Autodesk Inventor part; units mm, degrees
ref_plane "YZ Plane" through (0, 0, 0) normal (1, 0, 0) x (0, 1, 0)
ref_plane "XZ Plane" through (0, 0, 0) normal (0, 1, 0) x (-1, 0, 0)
ref_plane "XY Plane" through (0, 0, 0) normal (0, 0, 1) x (1, 0, 0)
sketch "Sketch1" plane through (0, 0, 0) normal (0, 0, 1) x (1, 0, 0)
  line L0 (-9, -62.5) -> (9, -62.5)
  line L1 (9, -62.5) -> (9, 62.5)
  line L2 (9, 62.5) -> (-9, 62.5)
  line L3 (-9, 62.5) -> (-9, -62.5)
  line L4 (-9, -62.5) -> (9, 62.5) construction
  line L5 (9, -62.5) -> (-9, 62.5) construction
  point P0 (0, 0)
  dimension "d0" = 18
  dimension "d1" = 125
extrude "Plate1" add sketch "Sketch1" along normal blind 2
sketch "Sketch2" plane through (-9, 60.5, 0) normal (0, 1, 0) x (-1, 0, 0)
  line L0 (-18, 0) -> (0, 0)
  line L1 (0, 0) -> (0, 25)
  line L2 (0, 25) -> (-18, 25)
  line L3 (-18, 25) -> (-18, 0)
edge flange "Flange1" height 25 angle 90 thickness 2 bend radius 2 thickness toward (0, 1, 0) relief tear relief width 2 relief depth 1 edges at (0, 62.5, 2) wall of the first edge with corners at (9, 60.5, 0) (-9, 60.5, 0) (-9, 60.5, 25) (9, 60.5, 25)
bend "Bend1"
corner "Corner1"
sketch "Sketch3" plane through (0, 0, 2) normal (0, 0, 1) x (1, 0, 0)
  line L0 (-1.75, -57.5) -> (1.75, -57.5) construction
  line L1 (-1.75, -59.2) -> (1.75, -59.2)
  line L2 (1.75, -55.8) -> (-1.75, -55.8)
  arc A0 (-1.75, -55.8) -> (-1.75, -59.2) centre (-1.75, -57.5) ccw
  arc A1 (1.75, -59.2) -> (1.75, -55.8) centre (1.75, -57.5) ccw
  line L3 (-1.75, 36.5) -> (1.75, 36.5) construction
  line L4 (-9, -62.5) -> (-9, 58.5)
  line L5 (-1.75, 34.8) -> (1.75, 34.8)
  line L6 (1.75, 38.2) -> (-1.75, 38.2)
  arc A2 (-1.75, 38.2) -> (-1.75, 34.8) centre (-1.75, 36.5) ccw
  arc A3 (1.75, 34.8) -> (1.75, 38.2) centre (1.75, 36.5) ccw
  line L7 (9, -62.5) -> (-9, -62.5)
  point P0 (0, 0)
  point P1 (0, -57.5)
  point P2 (0, 36.5)
  dimension "d13" = 94
  dimension "d14" = 5
  dimension "d15" = 3.4
  dimension "d16" = 3.5
extrude "Cut1" cut sketch "Sketch3" against normal blind 2
sketch "Sketch4" plane through (-9, 62.5, 25) normal (0, 1, 0) x (1, 0, 0)
  line L0 (12, 10.5) -> (6, 10.5) construction
  line L1 (12, 13.25) -> (6, 13.25)
  line L2 (6, 7.75) -> (12, 7.75)
  arc A0 (12, 7.75) -> (12, 13.25) centre (12, 10.5) ccw
  arc A1 (6, 13.25) -> (6, 7.75) centre (6, 10.5) ccw
  line L3 (18, 21) -> (18, 0)
  point P0 (9, 25)
  point P1 (9, 10.5)
  point P2 (18, 10.5)
  dimension "d19" = 5.5
  dimension "d20" = 6
extrude "Cut2" cut sketch "Sketch4" against normal blind 2
fillet "Fillet1" radius 4 4 edges at (-9, 61.5, 25) (9, 61.5, 25) (-9, -62.5, 1) (9, -62.5, 1)
equation "\"d17\" = Thickness"
equation "\"d21\" = Thickness"
equation "\"d2\" = Thickness"
equation "\"d3\" = BendReliefWidth"
equation "\"d4\" = BendReliefDepth"
equation "\"d5\" = MinimumRemnant"
equation "\"d6\" = TransitionRadius"
equation "\"d9\" = BendRadius"
equation "\"d10\" = CornerReliefSize"
equation "\"d11\" = GapSize"
equation "\"d12\" = JacobiRadiusSize"
equation "\"BendRadius\" = Thickness"
equation "\"BendReliefWidth\" = Thickness"
equation "\"BendReliefDepth\" = 0.5 * Thickness"
equation "\"CornerReliefSize\" = 4 * Thickness"
equation "\"MinimumRemnant\" = 2 * Thickness"
equation "\"TransitionRadius\" = BendRadius"
equation "\"JacobiRadiusSize\" = BendRadius"
equation "\"GapSize\" = Thickness"
properties part number "BREEZE-M30"
Model file for the job. Use its own axes, mm. A direction names the side the tool comes from. Give positions to 0.01 mm unless a question says otherwise; leave off trailing zeros. Order: outer loops, then holes, each group sorted by start corner. A loop starts at its lowest first (then second) coordinate and runs counter-clockwise, first axis right, second up. Notation, with made-up numbers: (42.25, -26) - (79.25, -26) arc R22 ccw to (79.25, 10) - close; hole circle Ø9 at (3, -27.75). An arc over 180 degrees is marked (long way). Write item = value, one per line. Start each with the question number.
1. Cut at A-A, the plane z = 14.5. List the corners of the cut face in (x, y), and give its area (3 significant figures).
2. Cut at B-B, the plane x = 0. List the corners of the cut face in (y, z), and give its area (3 significant figures).
3. Probe line 1 along Y through (x, z) = (-0.25, 23); line 2 along Z through (x, y) = (1.5, -7.5). List the from-to ranges inside material, lowest first.
4. Two-plate mould, pull along Z, no slides. Class faces 6 (the flat face through (0, -1, 0)), 7 (the cylindrical face through (7.797, 61.514, 23.859)), 8 (the cylindrical face through (-7.859, -61.297, 1.014)), 9 (the flat face through (0, 62, 17.25)): pulls with the +Z half, pulls with the -Z half, needs draft (parallel to the pull), parting line crosses it, or undercut.
5. Cut at C-C, the plane y = 36.5. List the corners of the cut face in (x, z).
6. Drop flat-ended pins along their axis: P1, Ø1.6, axis at x = -0.5, z = 1, coming from the +Y side; P2, Ø1.5, axis at x = -1, y = 3.5, coming from the +Z side; P3, Ø12, axis at y = -45, z = 13.5, coming from the -X side; P4, Ø5.5, axis at x = -2, z = 19.5, coming from the -Y side. Give the stop position or say it passes through.
7. Which spindle directions (+Z, -Z, +X, -X, +Y, -Y) get a long thin tool onto all of the face, cutting with end or side? Do faces 1 (the cylindrical face through (-7.859, 61.514, 23.797)), 2 (the flat face through (0, 60.5, 10)), 3 (the flat face through (0, 62, 11.75)), 4 (the cylindrical face through (-3.45, -57.46, 1.01)), 5 (the flat face through (0, 62.5, 10)). Say none if no direction does.
8. Cut at D-D, the plane y = -53. List the corners of the cut face in (x, z), and give its area (3 significant figures).
Taken from the geometry:
q1.outline = (-9, 60.5) - (-5.75, 60.5) - (-5.75, 62.5) - (-9, 62.5) - close; (5.75, 60.5) - (9, 60.5) - (9, 62.5) - (5.75, 62.5) - close
q1.area = 13.0 mm²
q2.outline = (-62.5, 0) - (-59.2, 0) - (-59.2, 2) - (-62.5, 2) - close; (-55.8, 0) - (34.8, 0) - (34.8, 2) - (-55.8, 2) - close; (38.2, 0) - (58.5, 0) arc R4 ccw to (62.5, 4) - (62.5, 11.75) - (60.5, 11.75) - (60.5, 4) arc R2 cw to (58.5, 2) - (38.2, 2) - close; (60.5, 17.25) - (62.5, 17.25) - (62.5, 25) - (60.5, 25) - close
q2.area = 269 mm²
q3.line_1 = 60.5 to 62.5
q3.line_2 = 0 to 2
q4.face_6 = pulls with the -Z half
q4.face_7 = pulls with the +Z half
q4.face_8 = needs draft
q4.face_9 = undercut
q5.outline = (-9, 0) - (-3.45, 0) - (-3.45, 2) - (-9, 2) - close; (3.45, 0) - (9, 0) - (9, 2) - (3.45, 2) - close
q6.P1 = 61.84
q6.P2 = 2
q6.P3 = through
q6.P4 = 60.5
q7.face_1 = +Z, -X, +Y, -Y
q7.face_2 = +Z, +X, -X, -Y
q7.face_3 = +Y, -Y
q7.face_4 = +Z, -Z
q7.face_5 = +Z, -Z, +X, -X, +Y
q8.outline = (-9, 0) - (9, 0) - (9, 2) - (-9, 2) - close
q8.area = 36.0 mm²
